The figure shows three views and two pictorial views of one solid part (mm, origin at its lowest corner). Answer the questions. A direction names the side the tool comes from. Coordinates: 2 decimals unless noted, no trailing zeros. Loops run counter-clockwise (first coordinate to the right, second up) from the corner with the lowest first, then second, coordinate; pieces in that order, holes last. Notation, with made-up numbers: M 11,64.25 L 43,64.25 A12 cw 43,77.25 Z; hole C -38,25.25 d3. An arc over 180 degrees is marked long. Return JSON: item names as keys, results as strings. Group by question number.
1. Given P1, Ø4, axis at y = 5, z = 7.5, coming from the -X side; P2, Ø2, axis at x = 7.5, y = 8, coming from the -Z side; P3, Ø6, axis at y = 4.5, z = 22.5, coming from the -X side, each flat-ended and moving along its own axis, determine where each tip first touches the part or whether it passes through.
2. Straight lines are drawn through the part: L1, parallel to X at y = 8.5, z = 12.7 (3 decimals); L2, parallel to X at y = 7.5, z = 11; L3, parallel to Z at x = 12, y = 9.75. For each, find the intervals that lie inside material, in ascending order. Write a range as from..to.
3. Section D-D (y = 1.25) is taken. Write down the section's boundary in (x, z), then the cut area to 3 significant figures.
4. Which of the six approach directions +Z, -Z, +X, -X, +Y, -Y give full straight-line access (tool end or side, diameter ignored) to the marked faces 1 and 2?
5. Section C-C (y = 7.75) is taken. Write down the section's boundary in (x, z) (3 decimals), then the cut area to 3 significant figures.
6. Section A-A (x = 12.7) is taken. Write down the section's boundary in (y, z) (3 decimals), then the cut area to 3 significant figures.
7. Section B-B (z = 12.7) is taken. Write down the section's boundary in (x, y) (3 decimals).
8. The mould has two halves that part along Z. Classify the marked faces 3, 4, 5 and 6: pulls with the +Z half, pulls with the -Z half, needs draft (parallel to the pull), parting line crosses it, or undercut.
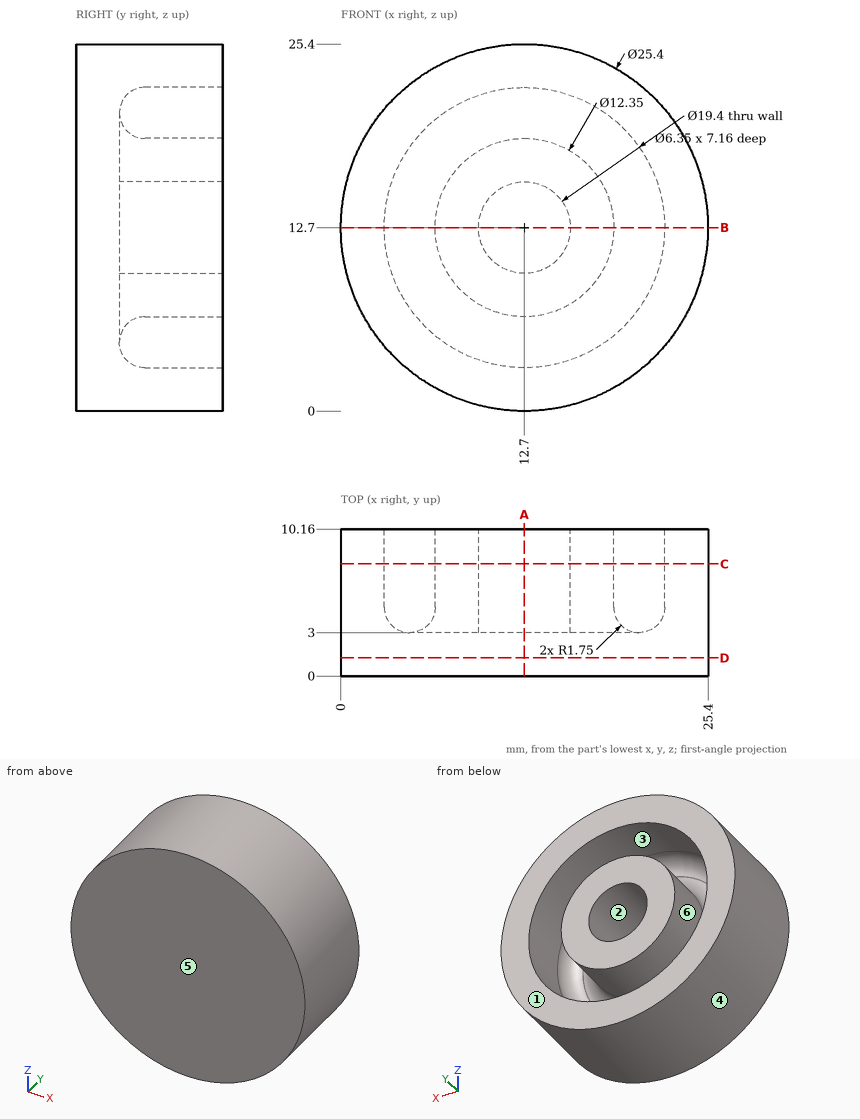
Worked out:
{
 "1": {"P1": "x = 0.41", "P2": "z = 0.71", "P3": "x = 1.97"},
 "2": {"L1": "0..3, 6.525..9.525, 15.875..18.875, 22.4..25.4", "L2": "0.11..3.15, 6.76..10.02, 15.38..18.64, 22.25..25.29", "L3": "0.02..3.03, 6.56..9.6, 15.8..18.84, 22.37..25.38"},
 "3": {"outline": "C 12.7,12.7 d25.4", "area": "507 mm^2"},
 "4": {"face 1": "+Z, -Z, +X, -X, +Y", "face 2": "+Y"},
 "5": {"outline": "C 12.7,12.7 d25.4; C 12.7,12.7 d12.35; hole C 12.7,12.7 d19.4; hole C 12.7,12.7 d6.35", "area": "299 mm^2"},
 "6": {"outline": "M 0,0 L 10.16,0 L 10.16,3 L 4.75,3 A1.75 cw 3,4.75 L 3,4.775 A1.75 cw 4.75,6.525 L 10.16,6.525 L 10.16,9.525 L 3,9.525 L 3,15.875 L 10.16,15.875 L 10.16,18.875 L 4.75,18.875 A1.75 cw 3,20.625 L 3,20.65 A1.75 cw 4.75,22.4 L 10.16,22.4 L 10.16,25.4 L 0,25.4 Z", "area": "165 mm^2"},
 "7": {"outline": "M 0,0 L 25.4,0 L 25.4,10.16 L 22.4,10.16 L 22.4,4.75 A1.75 cw 20.65,3 L 20.625,3 A1.75 cw 18.875,4.75 L 18.875,10.16 L 15.875,10.16 L 15.875,3 L 9.525,3 L 9.525,10.16 L 6.525,10.16 L 6.525,4.75 A1.75 cw 4.775,3 L 4.75,3 A1.75 cw 3,4.75 L 3,10.16 L 0,10.16 Z"},
 "8": {"face 3": "undercut", "face 4": "parting line crosses it", "face 5": "needs draft", "face 6": "undercut"}
}
